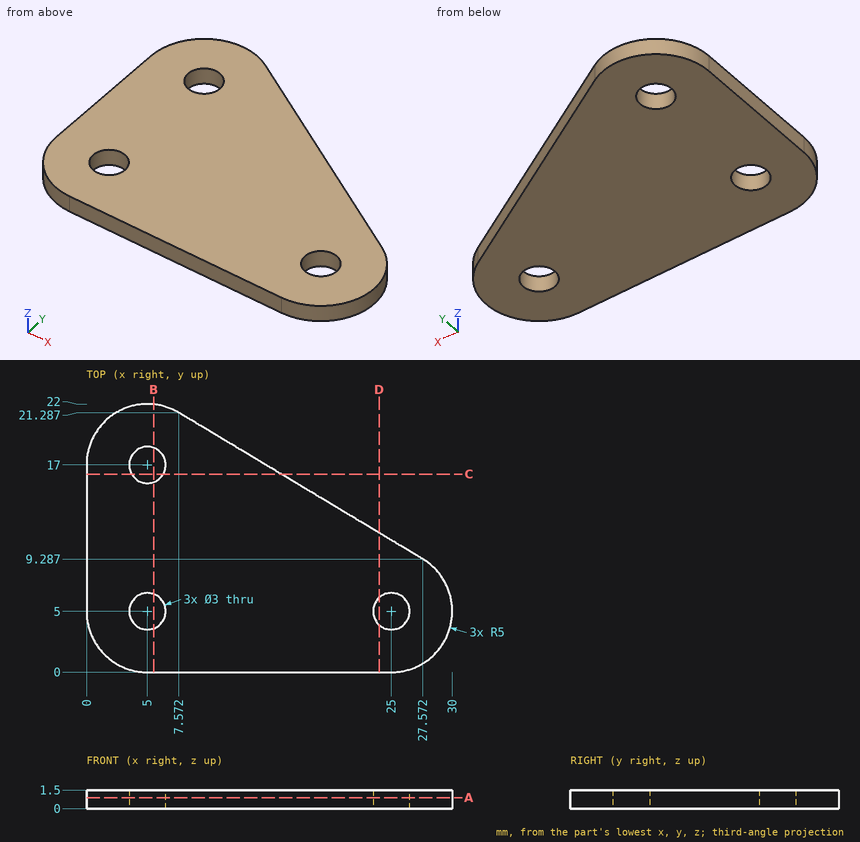
Answer from the drawing. Dimensions are ordinates in mm from the lowest x, y and z of the part. Coordinates: 2 decimals unless noted, no trailing zeros. Order: outer loops, then holes, each group sorted by start corner. A loop starts at its lowest first (then second) coordinate and runs counter-clockwise, first axis right, second up. Notation, with made-up numbers: (4, 50.5) - (17, 50.5) arc R19 cw to (17, 76.5) - close; hole circle Ø10 at (54, 29.25). An arc over 180 degrees is marked (long way). Put each result on its own line as item: value. Start each with the question number.
1) Find section A-A (z = 0.9). Give the vertices of the cut face in (x, y).
2) Find section D-D (x = 24). Give the vertices of the cut face in (y, z), plus the area to 3 significant figures.
3) Find the intervals of material crossed by line 1 (X direction, y = 5.5, z = 1.15) (1 decimal); line 2 (X direction, y = 4.25, z = 0.9) (1 decimal); line 3 (Y direction, x = 4, z = 1.25), in increasing order. Write a range as from..to.
4) Find section C-C (y = 16.25). Give the vertices of the cut face in (x, z).
5) Find section B-B (x = 5.5). Give the vertices of the cut face in (y, z) (1 decimal).
6) Flat-ended cylindrical pins translate along their axes: pin 1 (2.5 mm diameter, centred on x = 25, y = 5, fed in from +Z); pin 2 (4 mm diameter, centred on x = 5, y = 17, fed in from +Z). Find the tip coordinate at first contact, or state that the pin passes through.
Results list:
1. outline: (0, 5) arc R5 ccw to (5, 0) - (25, 0) arc R5 ccw to (27.57, 9.29) - (7.57, 21.29) arc R5 ccw to (0, 17) - close; hole circle Ø3 at (5, 5); hole circle Ø3 at (5, 17); hole circle Ø3 at (25, 5)
2. outline: (0, 0) - (3.88, 0) - (3.88, 1.5) - (0, 1.5) - close; (6.12, 0) - (11.43, 0) - (11.43, 1.5) - (6.12, 1.5) - close
2. area: 13.8 mm^2
3. line 1: x = 0..3.6, 6.4..23.6, 26.4..30
3. line 2: x = 0.1..3.7, 6.3..23.7, 26.3..29.9
3. line 3: y = 0.1..3.88, 6.12..15.88, 18.12..21.9
4. outline: (0, 0) - (3.7, 0) - (3.7, 1.5) - (0, 1.5) - close; (6.3, 0) - (15.97, 0) - (15.97, 1.5) - (6.3, 1.5) - close
5. outline: (0, 0) - (3.6, 0) - (3.6, 1.5) - (0, 1.5) - close; (6.4, 0) - (15.6, 0) - (15.6, 1.5) - (6.4, 1.5) - close; (18.4, 0) - (22, 0) - (22, 1.5) - (18.4, 1.5) - close
6. pin 1: passes through
6. pin 2: stops at z = 1.5
